Source: three-view drawing plus pictorial views. Frame: mm from the lowest corner of the part. Give positions to 0.01 mm unless a question says otherwise; leave off trailing zeros. Loops run counter-clockwise (first coordinate to the right, second up) from the corner with the lowest first, then second, coordinate; pieces in that order, holes last. Notation, with made-up numbers: (51, 80) -> (100, 80) arc R13 ccw to (100, 102) -> close; hole circle Ø8 at (25, 23.25). An arc over 180 degrees is marked (long way). Answer as a JSON object with one key per item and string values. Group by question number.
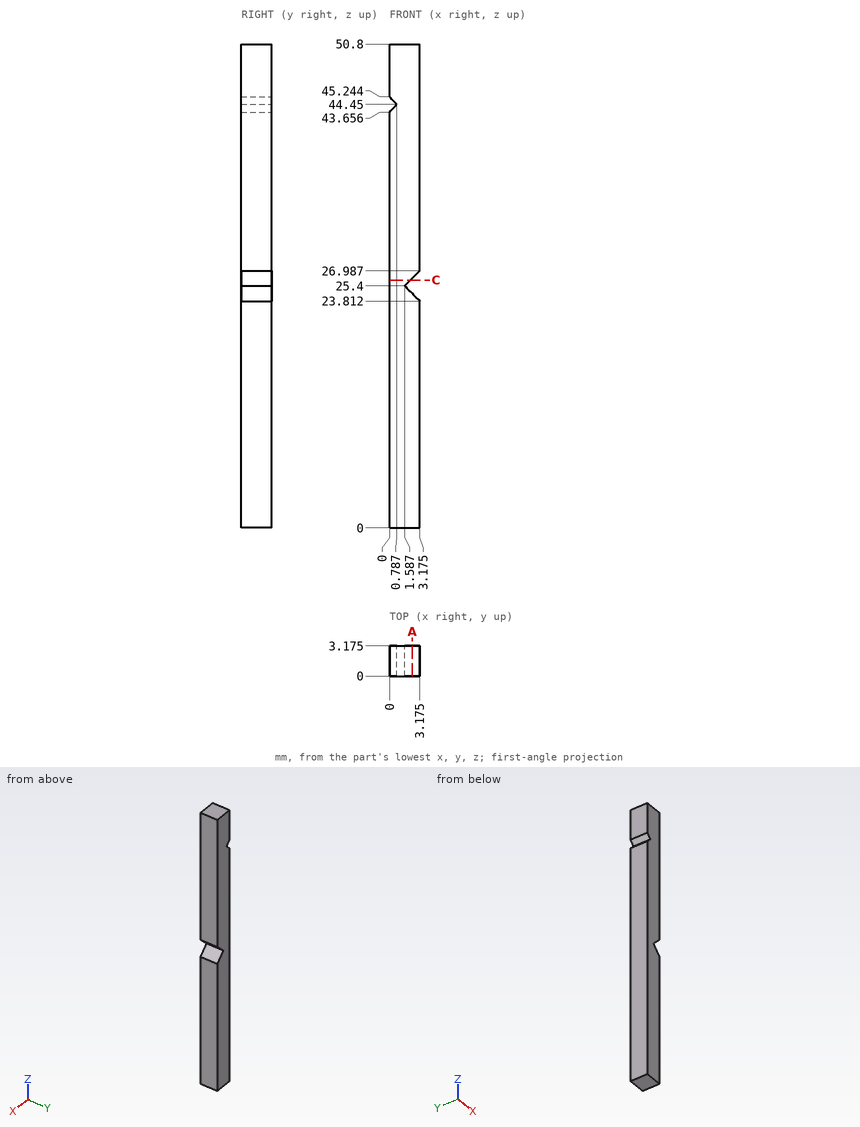
Q1. Section A-A on x = 2.4. Return the cut outline in (y, z) (1 decimal), then the cut area to 3 significant figures.
Q2. Ray query, probe 1 along Z at (x, y) = (0.7, 2.95) (1 decimal); probe 2 along Z at (x, y) = (2.05, 1.65) (1 decimal); probe 3 along X at (y, z) = (2.35, 25) (1 decimal). Return the intervals inside material, ascending.
Q3. Section C-C on z = 26. Return the cut outline in (x, y) (1 decimal).
Q4. Pin query (flat end, axial travel): pin 1 Ø1 at (y, z) = (2.5, 7.5) entering from -X. Return the tip coordinate at first contact, or that it passes through.
Numbers:
{
 "1": {"outline": "(0, 0) -> (3.2, 0) -> (3.2, 24.6) -> (0, 24.6) -> close; (0, 26.2) -> (3.2, 26.2) -> (3.2, 50.8) -> (0, 50.8) -> close", "area": "156 mm²"},
 "2": {"probe 1": "z = 0 to 44.4, 44.5 to 50.8", "probe 2": "z = 0 to 24.9, 25.9 to 50.8", "probe 3": "x = 0 to 2"},
 "3": {"outline": "(0, 0) -> (2.2, 0) -> (2.2, 3.2) -> (0, 3.2) -> close"},
 "4": {"pin 1": "stops at x = 0"}
}
